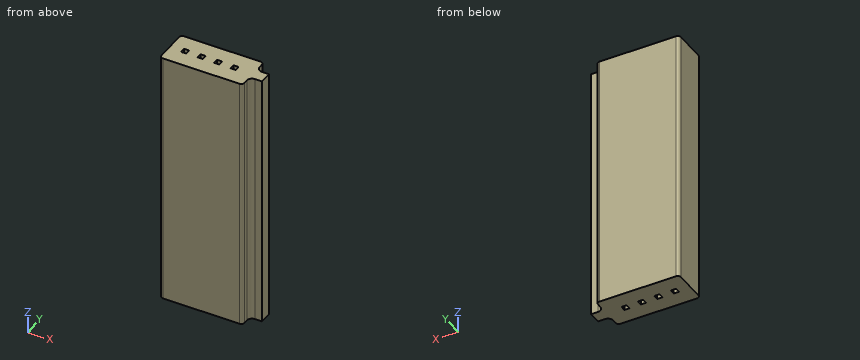
from build123d import *

# Parameters (mm, degrees)
BOSS_EXTRU_1_DEPTH         = 40
ESQUISSE3_W                = 0.8
ESQUISSE3_H                = 0.8
ENL_V_MAT_EXTRU_1_DEPTH    = 41.954853192
R_P_TITION_LIN_AIRE1_COUNT = 4
R_P_TITION_LIN_AIRE1_PITCH = 2.54
CONG_1_R                   = 0.8
CONG_2_R                   = 0.5


with BuildPart() as part:
    # Esquisse1 → Boss.-Extru.1 (new body)
    with BuildSketch(Plane.XY):
        Polygon((6.4, 0.95), (8.3, 0.95), (8.3, -0.95), (6.4, -0.95), (6.4, -2.9), (-6.4, -2.9), (-6.4, 2.9), (6.4, 2.9), align=None)
    extrude(amount=BOSS_EXTRU_1_DEPTH)

    # Esquisse3 → Enlèv. mat.-Extru.1 (cut, through all)
    with BuildSketch(Plane(origin=(0, 0, 0), x_dir=(-1, 0, 0), z_dir=(0, 0, -1))):
        with Locations((4.1, 0)):
            Rectangle(ESQUISSE3_W, ESQUISSE3_H)
    enl_v_mat_extru_1 = extrude(amount=-ENL_V_MAT_EXTRU_1_DEPTH, mode=Mode.SUBTRACT)

    # Répétition linéaire1: Enlèv. mat.-Extru.1 ×4
    with Locations(*[(i * R_P_TITION_LIN_AIRE1_PITCH, 0, 0) for i in range(1, R_P_TITION_LIN_AIRE1_COUNT)]):
        add(enl_v_mat_extru_1, mode=Mode.SUBTRACT)

    # Congé1
    cong_1_edges = [part.edges().sort_by_distance(p)[0] for p in [
        (6.4, 0.95, 20),
        (6.4, -0.95, 20),
    ]]
    fillet(cong_1_edges, radius=CONG_1_R)

    # Congé2
    cong_2_edges = [part.edges().sort_by_distance(p)[0] for p in [
        (6.4, -2.9, 20),
        (-6.4, -2.9, 20),
        (-6.4, 2.9, 20),
        (6.4, 2.9, 20),
    ]]
    fillet(cong_2_edges, radius=CONG_2_R)


solid = part.part
Work out the finished part from the listing and answer in its coordinate system (mm). Give positions to 0.01 mm unless a question says otherwise; leave off trailing zeros. Loops run counter-clockwise (first coordinate to the right, second up) from the corner with the lowest first, then second, coordinate; pieces in that order, holes last. Notation, with made-up numbers: (72.25, 28) -> (111.25, 28) arc R35 ccw to (111.25, 63) -> close; hole circle Ø11 at (16, -26). An arc over 180 degrees is marked (long way). Use a Markdown table: item, result. Add a question column.
1. Find the intervals of material crossed by probe 1 along Y at (x, z) = (3.25, 19.5); probe 2 along X at (y, z) = (2.3, 14); probe 3 along Y at (x, z) = (7.25, 33.5), in increasing order.
2. Section B-B on y = 1.4 is taken. Determine the outline of the cut face in (x, z), and give its area (3 significant figures).
3. Flat-ended cylindrical pins translate along their axes: pin 1 Ø0.7 at (y, z) = (2, 26) entering from +X; pin 2 Ø0.6 at (x, z) = (8, 28) entering from -Y. Find the tip coordinate at first contact, or state that the pin passes through.
4. Section C-C on y = -1.3 is taken. Determine the outline of the cut face in (x, z).
5. Section A-A on z = 16.5 is taken. State how many separate pieces and enclosed holes the cut face has, and give its area (4 significant figures).
Results below:
| question | item | result |
|---|---|---|
| 1 | probe 1 | y = -2.9 to -0.4, 0.4 to 2.9 |
| 1 | probe 2 | x = -6.4 to 6.4 |
| 1 | probe 3 | y = -0.95 to 0.95 |
| 2 | outline | (-6.4, 0) -> (6.48, 0) -> (6.48, 40) -> (-6.4, 40) -> close |
| 2 | area | 515 mm^2 |
| 3 | pin 1 | stops at x = 6.41 |
| 3 | pin 2 | stops at y = -0.95 |
| 4 | outline | (-6.4, 0) -> (6.54, 0) -> (6.54, 40) -> (-6.4, 40) -> close |
| 5 | separate pieces | 1 |
| 5 | enclosed holes | 4 |
| 5 | area | 75.35 mm^2 |
